Work out the finished part from the listing and answer in its coordinate system (mm). A direction names the side the tool comes from. Coordinates: 2 decimals unless noted, no trailing zeros. Write each loop counter-clockwise with the first axis right and the second up, starting at its lowest first coordinate (ties: lowest second). Pieces come first, ordered by that corner, then holes. Notation, with made-up numbers: M 25.5,8.5 L 60.5,8.5 A11 cw 60.5,26.5 Z; hole C -34.5,-3 d7. An arc over 180 degrees is marked long. Answer as CSV lines item,"result". Start each with the question number.
(1) A cutting plane is placed at A-A on z = 1.9. Give the vertices of the cut face in (x, y).
(2) A flat-ended cylindrical pin translates along its axis: P1, Ø1.5, axis at y = -24, z = 0.5, coming from the -X side. Find the tip coordinate at first contact, or state that the pin passes through.
(3) For faces 4 (the flat face through (0, 5, 5)), 5 (the flat face through (-1.5, 30, 2)), determine the directions among +Z, -Z, +X, -X, +Y, -Y from which every point of the face is accessible in a straight line to the end or side of a thin tool.
(4) Find the intervals of material crossed by L1, parallel to Y at x = 0, z = 2.75; L2, parallel to X at y = 28, z = 0.3; L3, parallel to X at y = 33.5, z = 2.75, in increasing order. Write a range as [from, to].
(5) The mould has two halves that part along X. Classify faces 1 (the flat face through (0, 5, 0)), 2 (the cylindrical face through (65.337, -20.576, 2.465)), 3 (the cylindrical face through (-1.5, -0.07, 2.46)): released by +X, released by -X, zero draft, split by the parting line, or undercut.
(6) A cutting plane is placed at C-C on x = -45.5. Give the vertices of the cut face in (y, z), then the cut area to 3 significant figures.
(7) A cutting plane is placed at D-D on y = 40. Give the vertices of the cut face in (x, z).
(8) A cutting plane is placed at B-B on y = -50. Give the vertices of the cut face in (x, z), then the cut area to 3 significant figures.
Solid Edge part; units mm, degrees
sketch "Sketch1" plane through (0, 0, 0) normal (0, 0, 1) x (1, 0, 0)
  line L0 (1.5, 54.9795) -> (1.5, 5.2915)
  arc A0 (1.5, 5.2915) -> (-1.5, 5.2915) centre (0, 0) ccw
  line L1 (-1.5, 5.2915) -> (-1.5, 54.9795)
  arc A1 (1.5, 54.9795) -> (-1.5, 54.9795) centre (0, 0) ccw
extrude "Protrusion1" add sketch "Sketch1" along normal blind 5
sketch "Sketch2" plane through (0, 0, 0) normal (0, 0, 1) x (1, 0, 0)
  circle A0 centre (0, 0) radius 5.5
  circle A1 centre (0, 0) radius 1.5
  circle A2 centre (0, 0) radius 55
  circle A3 centre (0, 0) radius 68.5
extrude "ExtrudedProtrusion_4" add sketch "Sketch2" along normal blind 5
Here are the results:
1,outline,"C 0,0 d137; hole C 0,0 d3; hole M -1.5,5.29 L -1.5,54.98 A55 ccw long 1.5,54.98 L 1.5,5.29 A5.5 cw long Z"
2,P1,"stops at x = -64.43"
3,face 4,"+Z, +X, -X, +Y, -Y"
3,face 5,"+Z, -Z"
4,L1,"y = [-68.5, -55], [-5.5, -1.5], [1.5, 68.5]"
4,L2,"x = [-62.52, -47.34], [-1.5, 1.5], [47.34, 62.52]"
4,L3,"x = [-59.75, -43.62], [-1.5, 1.5], [43.62, 59.75]"
5,face 1,"zero draft"
5,face 2,"split by the parting line"
5,face 3,"undercut"
6,outline,"M -51.21,0 L -30.9,0 L -30.9,5 L -51.21,5 Z; M 30.9,0 L 51.21,0 L 51.21,5 L 30.9,5 Z"
6,area,"203 mm^2"
7,outline,"M -55.61,0 L -37.75,0 L -37.75,5 L -55.61,5 Z; M -1.5,0 L 1.5,0 L 1.5,5 L -1.5,5 Z; M 37.75,0 L 55.61,0 L 55.61,5 L 37.75,5 Z"
8,outline,"M -46.82,0 L -22.91,0 L -22.91,5 L -46.82,5 Z; M 22.91,0 L 46.82,0 L 46.82,5 L 22.91,5 Z"
8,area,"239 mm^2"
